Geometry check sheet. Reference: the model listing, model coordinates, mm. A direction names the side the tool comes from. Round coordinates to 2 decimals unless told otherwise and drop trailing zeros. Order: outer loops, then holes, each group sorted by start corner. A loop starts at its lowest first (then second) coordinate and runs counter-clockwise, first axis right, second up. Notation, with made-up numbers: (-24, -4.75) -> (-2, -4.75) arc R31 cw to (-2, 33.25) -> close; hole circle Ø9 at (-27, -37.5). An arc over 180 degrees is marked (long way). Answer as a JSON object with one key per item and string values. Group by question number.
from build123d import *

# Parameters (mm, degrees)
SKETCH4_W           = 20
SKETCH4_H           = 70
BOSS_EXTRUDE2_DEPTH = 5
SKETCH5_W           = 7
SKETCH5_H           = 70
BOSS_EXTRUDE3_DEPTH = 10
SKETCH6_W           = 70
SKETCH6_H           = 1.998143523
CUT_EXTRUDE1_DEPTH  = 3
SKETCH8_W           = 10
SKETCH8_H           = 30
CUT_EXTRUDE2_DEPTH  = 74.484692283
FILLET3_START       = -1
FILLET3_DEPTH       = 6
FILLET3_2_DEPTH     = 5
FILLET4_R           = 5


with BuildPart() as part:
    # Sketch4 → Boss-Extrude2 (new body)
    with BuildSketch(Plane(origin=(0, 0, 0), x_dir=(1, 0, 0), z_dir=(0, 1, 0))):
        with Locations((10, 35)):
            Rectangle(SKETCH4_W, SKETCH4_H)
    extrude(amount=BOSS_EXTRUDE2_DEPTH)

    # Sketch5 → Boss-Extrude3 (add)
    with BuildSketch(Plane(origin=(0, 5, 0), x_dir=(1, 0, 0), z_dir=(0, 1, 0))):
        with Locations((3.5, 35)):
            Rectangle(SKETCH5_W, SKETCH5_H)
    extrude(amount=BOSS_EXTRUDE3_DEPTH)

    # Sketch6 → Cut-Extrude1 (cut)
    with BuildSketch(Plane(origin=(7, 0, 0), x_dir=(0, 0, -1), z_dir=(1, 0, 0))):
        with Locations((35, 10.999071762)):
            Rectangle(SKETCH6_W, SKETCH6_H)
    extrude(amount=-CUT_EXTRUDE1_DEPTH, mode=Mode.SUBTRACT)

    # Sketch8 → Cut-Extrude2 (cut, through all)
    with BuildSketch(Plane(origin=(0, 5, 0), x_dir=(1, 0, 0), z_dir=(0, 1, 0))):
        with Locations((15, 35)):
            Rectangle(SKETCH8_W, SKETCH8_H)
    extrude(amount=-CUT_EXTRUDE2_DEPTH, mode=Mode.SUBTRACT)

    # Fillet3: read off the stored shape, not the designer's step
    # Fillet3 outline → Fillet3 (cut)
    with BuildSketch(Plane(origin=(0, 0, 0), x_dir=(1, 0, 0), z_dir=(0, 1, 0)).offset(FILLET3_START)):
        with BuildLine():
            Line((20, 50), (20, 55))
            ThreePointArc((20, 55), (18.535533906, 51.464466094), (15, 50))
            Line((15, 50), (20, 50))
        make_face()
        with BuildLine():
            Line((20, 20), (15, 20))
            ThreePointArc((15, 20), (18.535533906, 18.535533906), (20, 15))
            Line((20, 15), (20, 20))
        make_face()
    extrude(amount=FILLET3_DEPTH, mode=Mode.SUBTRACT)

    # Fillet3 2 outline → Fillet3 2 (add)
    with BuildSketch(Plane(origin=(0, 0, 0), x_dir=(1, 0, 0), z_dir=(0, 1, 0))):
        with BuildLine():
            ThreePointArc((15, 20), (11.464466094, 21.464466094), (10, 25))
            Line((10, 25), (10, 20))
            Line((10, 20), (15, 20))
        make_face()
        with BuildLine():
            ThreePointArc((10, 45), (11.464466094, 48.535533906), (15, 50))
            Line((15, 50), (10, 50))
            Line((10, 50), (10, 45))
        make_face()
    extrude(amount=FILLET3_2_DEPTH)

    # Fillet4
    fillet4_edges = [part.edges().sort_by_distance(p)[0] for p in [
        (20, 2.5, -70),
        (20, 2.5, 0),
    ]]
    fillet(fillet4_edges, radius=FILLET4_R)


solid = part.part
Item 1: Sectioned sample at B-B, the plane y = 3. Enter the section's corners in (x, z), then the cut area to 3 significant figures.
Item 2: Sectioned sample at D-D, the plane x = 18. Enter the section's corners in (y, z).
Item 3: Mould release check, pull along Z, two halves, no side actions. Record for faces 1 (the flat face through (6, 6, 0)), 2 (the flat face through (6, 10, -35)), 3 (the flat face through (10, 3, -35)), 4 (the cylindrical face through (18, 3, -69)): pulls with the +Z half, pulls with the -Z half, needs draft (parallel to the pull), parting line crosses it, or undercut.
Item 4: Depth check by flat-ended pin: pin 1 Ø3.5 at (y, z) = (14, -36) entering from +X; pin 2 Ø2 at (y, z) = (4.5, -50.5) entering from +X; pin 3 Ø0.6 at (y, z) = (11, -41.5) entering from +X. Enter the tip coordinate at first touch or a pass-through.
Item 5: Thickness scan on L1, parallel to Y at x = 6, z = -16.5; L2, parallel to Z at x = 14.75, y = 3.75; L3, parallel to Y at x = 13.75, z = -56. Record the ranges inside material, lowest first.
Item 6: Sectioned sample at C-C, the plane z = -34. Enter the section's corners in (x, y).
Item 7: Set-up check for faces 5 (the flat face through (7, 7, -35)), 6 (the flat face through (0, 7, -35)), 7 (the flat face through (6, 11.998, -35)): record each of +Z, -Z, +X, -X, +Y, -Y from which the full face is reachable in a straight line by a thin tool's end or side.
Item 8: Sectioned sample at A-A, the plane x = 11. Enter the section's corners in (y, z).
Result:
{
 "1": {"outline": "(0, -70) -> (15, -70) arc R5 ccw to (20, -65) -> (20, -55) arc R5 ccw to (15, -50) arc R5 cw to (10, -45) -> (10, -25) arc R5 cw to (15, -20) arc R5 ccw to (20, -15) -> (20, -5) arc R5 ccw to (15, 0) -> (0, 0) -> close", "area": "1,090 mm2"},
 "2": {"outline": "(0, -69) -> (5, -69) -> (5, -51) -> (0, -51) -> close; (0, -19) -> (5, -19) -> (5, -1) -> (0, -1) -> close"},
 "3": {"face 1": "pulls with the +Z half", "face 2": "needs draft", "face 3": "undercut", "face 4": "pulls with the -Z half"},
 "4": {"pin 1": "stops at x = 7", "pin 2": "stops at x = 18.57", "pin 3": "stops at x = 4"},
 "5": {"L1": "y = 0 to 10, 12 to 15", "L2": "z = -70 to -49.99, -20.01 to 0", "L3": "y = 0 to 5"},
 "6": {"outline": "(0, 0) -> (10, 0) -> (10, 5) -> (7, 5) -> (7, 10) -> (4, 10) -> (4, 12) -> (7, 12) -> (7, 15) -> (0, 15) -> close"},
 "7": {"face 5": "+Z, -Z, +X, +Y", "face 6": "+Z, -Z, -X, +Y, -Y", "face 7": "+Z, -Z, +X"},
 "8": {"outline": "(0, -70) -> (5, -70) -> (5, -48) -> (0, -48) -> close; (0, -22) -> (5, -22) -> (5, 0) -> (0, 0) -> close"}
}
